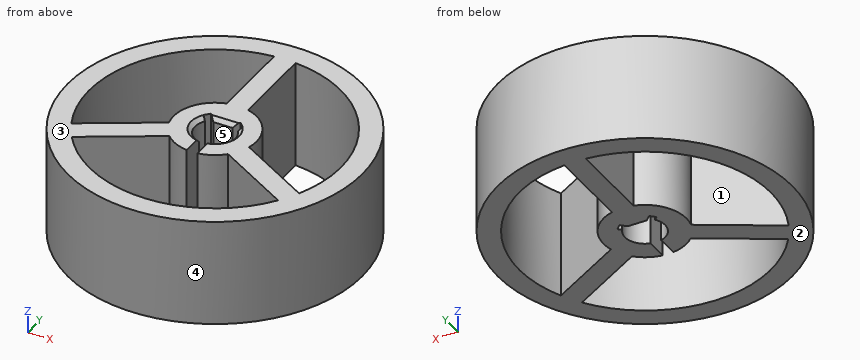
Autodesk Inventor part; units mm, degrees
ref_plane "YZ Plane" through (0, 0, 0) normal (1, 0, 0) x (0, 1, 0)
ref_plane "XZ Plane" through (0, 0, 0) normal (0, 1, 0) x (-1, 0, 0)
ref_plane "XY Plane" through (0, 0, 0) normal (0, 0, 1) x (1, 0, 0)
sketch "スケッチ1" plane through (0, 0, 0) normal (0, 0, 1) x (1, 0, 0)
  circle A0 centre (0, 0) radius 1.5
  circle A1 centre (0, 0) radius 3.1
  line L0 (-0.4, 0) -> (0.4, 0)
  line L1 (0.4, 0) -> (0.4, -3.1)
  line L2 (0.4, -3.1) -> (-0.4, -3.1)
  line L3 (-0.4, -3.1) -> (-0.4, 0)
  line L4 (-1.0712, 1.05) -> (1.0712, 1.05)
  circle A2 centre (0, 0) radius 11
  circle A3 centre (0, 0) radius 9.4
  line L5 (-1.4605, 1.0815) -> (-1.1105, 1.4385)
  line L6 (-1.1105, 1.4385) -> (0.175, 0.1785)
  line L7 (0.175, 0.1785) -> (-0.175, -0.1785)
  line L8 (-0.175, -0.1785) -> (-1.4605, 1.0815)
  line L9 (1.4605, 1.0815) -> (1.1105, 1.4385)
  line L10 (1.1105, 1.4385) -> (-0.175, 0.1785)
  line L11 (-0.175, 0.1785) -> (0.175, -0.1785)
  line L12 (0.175, -0.1785) -> (1.4605, 1.0815)
  line L13 (0, 0) -> (-1.0712, 1.05) construction
  line L14 (1.0712, 1.05) -> (0, 0) construction
  point P0 (0.4, -1.4457)
  point P1 (0.4, -3.0741)
  point P2 (-0.4, -3.0741)
  point P3 (-0.4, -1.4457)
  point P4 (-0.7141, 1.05)
  point P5 (0.7141, 1.05)
  point P6 (1.2312, 0.8568)
  point P7 (-1.2312, 0.8568)
  dimension "SHAFT_D" = 3
  dimension "SLIT" = 0.8
  dimension "HUB_THIN" = 1.6
  dimension "d3" = 1.05
  dimension "WHEEL_D" = 22
  dimension "d5" = 1.6
  dimension "d18" = 0.5
  dimension "d19" = 1.8
extrude "ハブ＆リム" add sketch "スケッチ1" along normal blind 8 contours A0 L12 L9 L10 L6 L5 L8 L3 A1 L1 | L10 L4 L6 A0 | A2
sketch "スケッチ2" plane through (0, 0, 0) normal (0, 0, 1) x (1, 0, 0)
  line L0 (-0.8, 2.6) -> (0.8, 2.6)
  line L1 (0.8, 2.6) -> (0.8, 9.4)
  line L2 (0.8, 9.4) -> (-0.8, 9.4)
  line L3 (-0.8, 9.4) -> (-0.8, 2.6)
  circle A0 centre (0, 0) radius 9.4
  point P0 (0, 9.4)
  dimension "d8" = 1.6
  dimension "d9" = 2.6
extrude "スポーク" add sketch "スケッチ2" along normal up to surface (8 mm away) contours L3 A0 L1 L0 | L3 L2 A0 | A0 L2 L1 picked at (0, 4.8667)
pattern_circular "円形状パターン1" count 3 over 360 about axis through (0, 0, -10) along (0, 0, 1) of "スポーク"
chamfer "面取り1" distance 0.3 angle 45 3 edges at (-1.4109, -0.5094, 8) (0, 1.05, 8) (1.4109, -0.5094, 8)
equation "\"d5\" = HUB_THIN"
properties part number "D-Shaft_Wheel3"
Can you work these out from the model? Positions are in its coordinate system, mm. Face numbers are marked on the shaded views. A direction names the side the tool comes from. Coordinates: 2 decimals unless noted, no trailing zeros. Order: outer loops, then holes, each group sorted by start corner. A loop starts at its lowest first (then second) coordinate and runs counter-clockwise, first axis right, second up. Notation, with made-up numbers: M 40.5,-14 L 76.5,-14 A21 ccw 76.5,17 Z; hole C -14,71.5 d2. An arc over 180 degrees is marked long. Write item = value, one per line.
(1) If we mould it in two halves opening along X, with no side actions, what happens to the marked faces 3, 4 and 5? For each: pulls with the +X half, pulls with the -X half, needs draft (parallel to the pull), parting line crosses it, or undercut.
Results are:
face_3 = needs draft
face_4 = parting line crosses it
face_5 = undercut
(2) Suppose I cut it at B-B on x = 0. Please give me the cut outline in (y, z), plus the area to 3 significant figures.
Results are:
outline = M -11,0 L -9.4,0 L -9.4,8 L -11,8 Z; M 1.05,0 L 11,0 L 11,8 L 1.35,8 L 1.05,7.7 Z
area = 92.4 mm2
(3) Suppose I cut it at D-D on x = 5. Please give me the cut outline in (y, z).
Results are:
outline = M -9.8,0 L -7.96,0 L -7.96,8 L -9.8,8 Z; M -3.81,0 L -1.96,0 L -1.96,8 L -3.81,8 Z; M 7.96,0 L 9.8,0 L 9.8,8 L 7.96,8 Z
(4) I need wall thicknesses on line 1 along X through (y, z) = (1.5, 6.5); line 2 along X through (y, z) = (-0.75, 6.5); line 3 along X through (y, z) = (2, 7.75). Which ranges of each line are inside material? Lowest first, please. Write a range as [from, to].
Results are:
line_1 = [-10.9, -9.28], [-2.71, 2.71], [9.28, 10.9]
line_2 = [-10.97, -9.37], [-3.01, -1.3], [1.3, 3.01], [9.37, 10.97]
line_3 = [-10.82, -9.18], [-2.37, 2.37], [9.18, 10.82]
(5) For the marked faces 1 and 2, which set-ups out of +Z, -Z, +X, -X, +Y, -Y let a thin tool reach every point of the face, with its end or its side?
Results are:
face_1 = +Z, -Z
face_2 = -Z, +X, -X, +Y, -Y
(6) Suppose I cut it at C-C on z = 6. State how many separate pieces and enclosed holes the cut face has, plus the area to 3 significant figures.
Results are:
separate_pieces = 1
enclosed_holes = 3
area = 155 mm2
(7) For pin 1 Ø1.9 at (y, z) = (4.5, 5) entering from +X; pin 2 Ø2 at (x, z) = (-8, 7) entering from +Y; pin 3 Ø0.5 at (y, z) = (-2, 4.5) entering from +X, each with a flat end and sliding along its axis, tell me the tip position at first contact or that it passes through.
Results are:
pin_1 = 10.41
pin_2 = 8.49
pin_3 = 10.86
(8) Suppose I cut it at A-A on y = 0. Please give me the cut outline in (x, z), plus the area to 3 significant figures.
Results are:
outline = M -11,0 L -9.4,0 L -9.4,8 L -11,8 Z; M -3.1,0 L -1.5,0 L -1.5,7.7 L -1.8,8 L -3.1,8 Z; M 1.5,0 L 3.1,0 L 3.1,8 L 1.8,8 L 1.5,7.7 Z; M 9.4,0 L 11,0 L 11,8 L 9.4,8 Z
area = 51.1 mm2
